from build123d import *

# Parameters (mm, degrees)
CROQUIS1_R              = 15
CROQUIS1_R_2            = 5
SALIENTE_EXTRUIR1_DEPTH = 16
CORTAR_EXTRUIR1_START   = -12
CROQUIS2_R              = 22
CROQUIS2_R_2            = 15
CORTAR_EXTRUIR1_DEPTH   = 12
CORTAR_EXTRUIR2_DEPTH   = 8
CROQUIS4_R              = 6
SALIENTE_EXTRUIR2_DEPTH = 14


with BuildPart() as part:
    # Croquis1 → Saliente-Extruir1 (new, symmetric)
    with BuildSketch(Plane.XY):
        Polygon((-23, 73), (23, 73), (48, 12), (48, 0), (-48, 0), (-48, 12), align=None)
        with Locations((0, 40)):
            Circle(CROQUIS1_R, mode=Mode.SUBTRACT)
        with Locations((0, 9)):
            Circle(CROQUIS1_R_2, mode=Mode.SUBTRACT)
    extrude(amount=SALIENTE_EXTRUIR1_DEPTH, both=True)

    # Croquis2 → Cortar-Extruir1 (cut)
    with BuildSketch(Plane.XY.offset(16).offset(CORTAR_EXTRUIR1_START)):
        with Locations((0, 40)):
            Circle(CROQUIS2_R)
        with Locations((0, 40)):
            Circle(CROQUIS2_R_2, mode=Mode.SUBTRACT)
    cortar_extruir1 = extrude(amount=CORTAR_EXTRUIR1_DEPTH, mode=Mode.SUBTRACT)

    # Croquis3 → Cortar-Extruir2 (cut)
    with BuildSketch(Plane.XY.offset(16)):
        Polygon((23, 73), (36.524590164, 40), (31.524590164, 40), (18, 73), align=None)
        Polygon((-18, 73), (-23, 73), (-36.524590164, 40), (-31.524590164, 40), align=None)
    cortar_extruir2 = extrude(amount=-CORTAR_EXTRUIR2_DEPTH, mode=Mode.SUBTRACT)

    # Simetría1: Cortar-Extruir1, Cortar-Extruir2 across plane
    add(cortar_extruir1.mirror(Plane.XY), mode=Mode.SUBTRACT)
    add(cortar_extruir2.mirror(Plane.XY), mode=Mode.SUBTRACT)

    # Croquis4 → Saliente-Extruir2 (add, symmetric)
    with BuildSketch(Plane(origin=(0, 0, 0), x_dir=(0, 0, -1), z_dir=(1, 0, 0))):
        with BuildLine():
            Line((-12, 73), (12, 73))
            Line((12, 73), (12, 86))
            ThreePointArc((12, 86), (0, 98), (-12, 86))
            Line((-12, 86), (-12, 73))
        make_face()
        with Locations((0, 86)):
            Circle(CROQUIS4_R, mode=Mode.SUBTRACT)
    extrude(amount=SALIENTE_EXTRUIR2_DEPTH, both=True)


solid = part.part
Work out the finished part from the listing and answer in its coordinate system (mm). A direction names the side the tool comes from. Give positions to 0.01 mm unless a question says otherwise; leave off trailing zeros. Write each loop counter-clockwise with the first axis right and the second up, starting at its lowest first coordinate (ties: lowest second). Pieces come first, ordered by that corner, then holes.
Q1. The part is cut by section D-D on x = -39.5. Give the vertices of the cut face in (y, z), and give its area (3 significant figures).
Answer:
outline: (0, -16) - (32.74, -16) - (32.74, 16) - (0, 16) - close
area: 1,050 mm2
Q2. The part is cut by section A-A on z = 0. Give the vertices of the cut face in (x, y).
Answer:
outline: (-48, 0) - (48, 0) - (48, 12) - (23, 73) - (14, 73) - (14, 80) - (-14, 80) - (-14, 73) - (-23, 73) - (-48, 12) - close; (-14, 92) - (14, 92) - (14, 98) - (-14, 98) - close; hole circle Ø30 at (0, 40); hole circle Ø10 at (0, 9)
Q3. Given pin 1 (22 mm diameter, centred on x = -6, y = 49, fed in from +Z); pin 2 (2.5 mm diameter, centred on x = 33.5, z = -13, fed in from +Y); pin 3 (19 mm diameter, centred on y = 83, z = -3, fed in from -X); pin 4 (18 mm diameter, centred on x = 0, y = 40, fed in from +Z), each flat-ended and moving along its own axis, determine where each tip first touches the part or whether it passes through.
Answer:
pin 1: stops at z = 4
pin 2: stops at y = 40
pin 3: stops at x = -14
pin 4: passes through
Q4. A tool of negligible diameter and unlimited length cuts with its end or side. For faces 1 (the face through (14, 80, -2)), 2 (the face through (0, 80, 12)), 3 (the face through (34, 40, 12)), 4 (the face through (27, 57, -8)), from which of +Z, -Z, +X, -X, +Y, -Y can it reach the whole face along a straight path? Write none if from no direction.
Answer:
face 1: +Z, -Z, +X, +Y
face 2: +Z, +X, -X, +Y
face 3: +Z, +X, +Y
face 4: -Z, +X, +Y
Q5. The part is cut by section C-C on y = 45. Give the vertices of the cut face in (x, z).
Answer:
outline: (-34.48, -8) - (-29.48, -8) - (-29.48, -16) - (-21.42, -16) - (-21.42, -4) - (-14.14, -4) - (-14.14, 4) - (-21.42, 4) - (-21.42, 16) - (-29.48, 16) - (-29.48, 8) - (-34.48, 8) - close; (14.14, -4) - (21.42, -4) - (21.42, -16) - (29.48, -16) - (29.48, -8) - (34.48, -8) - (34.48, 8) - (29.48, 8) - (29.48, 16) - (21.42, 16) - (21.42, 4) - (14.14, 4) - close
Q6. The part is cut by section B-B on x = 7. Give the vertices of the cut face in (y, z).
Answer:
outline: (0, -16) - (19.14, -16) - (19.14, -4) - (26.73, -4) - (26.73, 4) - (19.14, 4) - (19.14, 16) - (0, 16) - close; (53.27, -4) - (60.86, -4) - (60.86, -16) - (73, -16) - (73, -12) - (86, -12) arc R12 ccw to (86, 12) - (73, 12) - (73, 16) - (60.86, 16) - (60.86, 4) - (53.27, 4) - close; hole circle Ø12 at (86, 0)
Q7. For a pull along Y with two mould halves and no side action, classify faces 5 (the face through (34, 40, -12)), 6 (the face through (-1.953, 54.872, -0.056)), 7 (the face through (48, 6, 0)) as released by +Y, released by -Y, zero draft, split by the parting line, or undercut.
Answer:
face 5: released by +Y
face 6: undercut
face 7: zero draft
Q8. Straight lines are drawn through the part: L1, parallel to Y at x = 0, z = 13.25; L2, parallel to Y at x = -1, z = -14; L3, parallel to Y at x = 3, z = 1. For each, find the intervals that lie inside material, in ascending order.
Answer:
L1: y = 0 to 4, 14 to 18, 62 to 73
L2: y = 0 to 4.1, 13.9 to 18.02, 61.98 to 73
L3: y = 0 to 5, 13 to 25.3, 54.7 to 80.08, 91.92 to 97.96
